Source: CAD feature listing. Evaluate the final solid. Frame: model axes, mm. A direction names the side the tool comes from. Coordinates: 2 decimals unless noted, no trailing zeros. Order: outer loops, then holes, each group sorted by start corner. A loop starts at its lowest first (then second) coordinate and runs counter-clockwise, first axis right, second up. Notation, with made-up numbers: (-8, 39) -> (14, 39) arc R26 ccw to (14, 56) -> close; hole circle Ø9 at (-19, 47). An arc over 180 degrees is marked (long way). Put each result on its own line as item: value.
from build123d import *

# Parameters (mm, degrees)
SKETCH1_W               = 535
SKETCH1_H               = 395
BOSS_EXTRUDE1_DEPTH     = 3
SKETCH2_W               = 105
SKETCH2_H               = 75
CUT_EXTRUDE1_DEPTH      = 3
MIRROR2_COPY_1_SKETCH_W = 105
MIRROR2_COPY_1_SKETCH_H = 75
MIRROR2_COPY_1_DEPTH    = 3
SKETCH3_W               = 3
SKETCH3_H               = 245
BOSS_EXTRUDE2_DEPTH     = 90
SKETCH4_W               = 245
SKETCH4_H               = 3
BOSS_EXTRUDE3_DEPTH     = 25
SKETCH5_W               = 3
SKETCH5_H               = 245
BOSS_EXTRUDE4_DEPTH     = 90
SKETCH6_W               = 245
SKETCH6_H               = 3
BOSS_EXTRUDE5_DEPTH     = 10
SKETCH7_R               = 1.5
CUT_EXTRUDE2_DEPTH      = 3
SKETCH8_R               = 1.5
CUT_EXTRUDE3_DEPTH      = 4
SKETCH9_R               = 1.5
CUT_EXTRUDE4_DEPTH      = 4


with BuildPart() as part:
    # Sketch1 → Boss-Extrude1 (new body)
    with BuildSketch(Plane(origin=(0, 0, 0), x_dir=(1, 0, 0), z_dir=(0, 1, 0))):
        Rectangle(SKETCH1_W, SKETCH1_H)
    extrude(amount=BOSS_EXTRUDE1_DEPTH)

    # Sketch2 → Cut-Extrude1 (cut)
    with BuildSketch(Plane(origin=(0, 3, 0), x_dir=(1, 0, 0), z_dir=(0, 1, 0))):
        with Locations((-215, 160)):
            Rectangle(SKETCH2_W, SKETCH2_H)
    cut_extrude1 = extrude(amount=-CUT_EXTRUDE1_DEPTH, mode=Mode.SUBTRACT)

    # Mirror1: Cut-Extrude1 across plane
    add(cut_extrude1.mirror(Plane.XY), mode=Mode.SUBTRACT)

    # Mirror2: Cut-Extrude1 across plane
    add(cut_extrude1.mirror(Plane(origin=(0, 0, 0), x_dir=(0, 0, 1), z_dir=(1, 0, 0))), mode=Mode.SUBTRACT)

    # Mirror2 copy 1 sketch → Mirror2 copy 1 (cut)
    with BuildSketch(Plane(origin=(0, 3, 0), x_dir=(-1, 0, 0), z_dir=(0, 1, 0))):
        with Locations((-215, 160)):
            Rectangle(MIRROR2_COPY_1_SKETCH_W, MIRROR2_COPY_1_SKETCH_H)
    extrude(amount=-MIRROR2_COPY_1_DEPTH, mode=Mode.SUBTRACT)

    # Sketch3 → Boss-Extrude2 (add)
    with BuildSketch(Plane(origin=(0, 3, 0), x_dir=(1, 0, 0), z_dir=(0, 1, 0))):
        with Locations((-266, 0)):
            Rectangle(SKETCH3_W, SKETCH3_H)
    extrude(amount=BOSS_EXTRUDE2_DEPTH)

    # Sketch4 → Boss-Extrude3 (add)
    with BuildSketch(Plane(origin=(-264.5, 0, 0), x_dir=(0, 0, -1), z_dir=(1, 0, 0))):
        with Locations((0, 91.5)):
            Rectangle(SKETCH4_W, SKETCH4_H)
    extrude(amount=BOSS_EXTRUDE3_DEPTH)

    # Sketch5 → Boss-Extrude4 (add)
    with BuildSketch(Plane(origin=(0, 3, 0), x_dir=(1, 0, 0), z_dir=(0, 1, 0))):
        with Locations((266, 0)):
            Rectangle(SKETCH5_W, SKETCH5_H)
    extrude(amount=BOSS_EXTRUDE4_DEPTH)

    # Sketch6 → Boss-Extrude5 (add)
    with BuildSketch(Plane.ZY.offset(-264.5)):
        with Locations((0, 91.5)):
            Rectangle(SKETCH6_W, SKETCH6_H)
    extrude(amount=BOSS_EXTRUDE5_DEPTH)

    # Sketch7 → Cut-Extrude2 (cut)
    with BuildSketch(Plane(origin=(0, 3, 0), x_dir=(1, 0, 0), z_dir=(0, 1, 0))):
        with Locations((0, 50)):
            Circle(SKETCH7_R)
        with Locations((0, -50)):
            Circle(SKETCH7_R)
    extrude(amount=-CUT_EXTRUDE2_DEPTH, mode=Mode.SUBTRACT)

    # Sketch8 → Cut-Extrude3 (cut, through all)
    with BuildSketch(Plane(origin=(0, 3, 0), x_dir=(1, 0, 0), z_dir=(0, 1, 0))):
        with Locations((0, -190.5)):
            Circle(SKETCH8_R)
    cut_extrude3 = extrude(amount=-CUT_EXTRUDE3_DEPTH, mode=Mode.SUBTRACT)

    # Sketch9 → Cut-Extrude4 (cut, through all)
    with BuildSketch(Plane(origin=(0, 3, 0), x_dir=(1, 0, 0), z_dir=(0, 1, 0))):
        with Locations((0, -115.5)):
            Circle(SKETCH9_R)
    cut_extrude4 = extrude(amount=-CUT_EXTRUDE4_DEPTH, mode=Mode.SUBTRACT)

    # Mirror3: Cut-Extrude3, Cut-Extrude4 across plane
    add(cut_extrude3.mirror(Plane.XY), mode=Mode.SUBTRACT)
    add(cut_extrude4.mirror(Plane.XY), mode=Mode.SUBTRACT)


solid = part.part
1. First-contact query: pin 1 (3.5 mm diameter, centred on x = 0, z = 115.5, fed in from +Y); pin 2 (3.5 mm diameter, centred on y = 1, z = 149.5, fed in from +X); pin 3 (2.5 mm diameter, centred on y = 1.5, z = 145, fed in from -X). Flat tips, straight axial feed; report the tip coordinate or a pass-through.
Numbers:
pin 1: stops at y = 3
pin 2: stops at x = 162.5
pin 3: stops at x = -162.5
2. Set-up query: faces 4 (the flat face through (266, 26, 122.5)), 5 (the flat face through (-266, 33, 122.5)), 6 (the flat face through (266, 26, -122.5)), 7 (the flat face through (-266, 33, -122.5)), 8 (the flat face through (-264.5, 46, 2)). Return all of +Z, -Z, +X, -X, +Y, -Y with unobstructed straight access to the full face (end or side cutting, diameter ignored); none if empty.
Numbers:
face 4: +Z, +X, +Y, -Y
face 5: +Z, -X, +Y, -Y
face 6: -Z, +X, +Y, -Y
face 7: -Z, -X, +Y, -Y
face 8: +Z, -Z
3. Pull-direction query (Y, two-part tool) for faces 1 (the flat face through (-254, 93, 2)), 2 (the flat face through (-4, 0, -3)), 3 (the flat face through (-252, 90, 2)); classes: pulls with the +Y half, pulls with the -Y half, needs draft (parallel to the pull), parting line crosses it, or undercut.
Numbers:
face 1: pulls with the +Y half
face 2: pulls with the -Y half
face 3: undercut
4. Cut plane C-C on x = 204.5. Output: boundary loops of the cut face in (y, z), plus the area to 3 significant figures.
Numbers:
outline: (0, -122.5) -> (3, -122.5) -> (3, 122.5) -> (0, 122.5) -> close
area: 735 mm2
5. Ray query, line 1 along X through (y, z) = (0.75, 115.5); line 2 along X through (y, z) = (26, 22); line 3 along Y through (x, z) = (-125, 9.5). Return the intervals inside material, ascending.
Numbers:
line 1: x = -267.5 to -1.5, 1.5 to 267.5
line 2: x = -267.5 to -264.5, 264.5 to 267.5
line 3: y = 0 to 3
6. Cut plane D-D on z = 145.5. Output: boundary loops of the cut face in (x, y).
Numbers:
outline: (-162.5, 0) -> (162.5, 0) -> (162.5, 3) -> (-162.5, 3) -> close
7. Cut plane B-B on z = 11. Output: boundary loops of the cut face in (x, y), plus the area to 3 significant figures.
Numbers:
outline: (-267.5, 0) -> (267.5, 0) -> (267.5, 93) -> (254.5, 93) -> (254.5, 90) -> (264.5, 90) -> (264.5, 3) -> (-264.5, 3) -> (-264.5, 90) -> (-239.5, 90) -> (-239.5, 93) -> (-267.5, 93) -> close
area: 2,250 mm2
8. Cut plane A-A on y = 44. Output: boundary loops of the cut face in (x, z), plus the area to 3 significant figures.
Numbers:
outline: (-267.5, -122.5) -> (-264.5, -122.5) -> (-264.5, 122.5) -> (-267.5, 122.5) -> close; (264.5, -122.5) -> (267.5, -122.5) -> (267.5, 122.5) -> (264.5, 122.5) -> close
area: 1,470 mm2
